Check sheet for the modelled part. Datum: model origin and axes. Units: mm. Give positions to 0.01 mm unless a question says otherwise; leave off trailing zeros. Loops run counter-clockwise (first coordinate to the right, second up) from the corner with the lowest first, then second, coordinate; pieces in that order, holes last.
```python
from build123d import *

# Parameters (mm, degrees)
F0_R     = 1.5
F0_R_2   = 1.25
F0_R_3   = 3.35
F1_DEPTH = 2.5


with BuildPart() as f1:
    # F0 (on Top) → F1 (new body)
    with BuildSketch(Plane.XY):
        with BuildLine():
            Line((-8.0347370397, 15.957047836), (-11, -56))
            Line((-11, -56), (-7.9966708881, -63.1295586577))
            ThreePointArc((-7.9966708881, -63.1295586577), (0, -68), (7.9966708881, -63.1295586577))
            Line((7.9966708881, -63.1295586577), (11, -56))
            Line((11, -56), (8.0347370397, 15.957047836))
            ThreePointArc((8.0347370397, 15.957047836), (8.1132286629, 16.7731349004), (8.4097212043, 17.5374981677))
            Line((8.4097212043, 17.5374981677), (12.5735371817, 25.0323669271))
            ThreePointArc((12.5735371817, 25.0323669271), (12.8772178164, 25.8277582971), (12.9452230888, 26.6764305791))
            Line((12.9452230888, 26.6764305791), (12.0626597761, 40.7974435824))
            ThreePointArc((12.0626597761, 40.7974435824), (11.8483082239, 41.738438851), (11.3462718477, 42.5626828443))
            Line((11.3462718477, 42.5626828443), (6.8979650397, 47.7523741204))
            ThreePointArc((6.8979650397, 47.7523741204), (5.8737656612, 48.5255386955), (4.6201952326, 48.8))
            Line((4.6201952326, 48.8), (-4.6201952326, 48.8))
            ThreePointArc((-4.6201952326, 48.8), (-5.8737656612, 48.5255386955), (-6.8979650397, 47.7523741204))
            Line((-6.8979650397, 47.7523741204), (-11.3462718477, 42.5626828443))
            ThreePointArc((-11.3462718477, 42.5626828443), (-11.8483082239, 41.738438851), (-12.0626597761, 40.7974435824))
            Line((-12.0626597761, 40.7974435824), (-12.9452230888, 26.6764305791))
            ThreePointArc((-12.9452230888, 26.6764305791), (-12.8772178164, 25.8277582971), (-12.5735371817, 25.0323669271))
            Line((-12.5735371817, 25.0323669271), (-8.4097212043, 17.5374981677))
            ThreePointArc((-8.4097212043, 17.5374981677), (-8.1132286629, 16.7731349004), (-8.0347370397, 15.957047836))
        make_face()
        with Locations((-6, -57.6)):
            Circle(F0_R, mode=Mode.SUBTRACT)
        with Locations((-6, -47.6)):
            Circle(F0_R, mode=Mode.SUBTRACT)
        with Locations((6, -57.6)):
            Circle(F0_R, mode=Mode.SUBTRACT)
        with Locations((6, -47.6)):
            Circle(F0_R, mode=Mode.SUBTRACT)
        with Locations((0, 1.25)):
            Circle(F0_R_2, mode=Mode.SUBTRACT)
        with Locations((0, 8.75)):
            Circle(F0_R_2, mode=Mode.SUBTRACT)
        with BuildLine():
            Line((-7.9549512883, 26.8285010896), (-5.6922095886, 29.0912427894))
            ThreePointArc((-5.6922095886, 29.0912427894), (-3.3587572106, 29.0912427894), (-3.3587572106, 26.7577904114))
            Line((-3.3587572106, 26.7577904114), (-5.6214989104, 24.4950487117))
            ThreePointArc((-5.6214989104, 24.4950487117), (-7.9549512883, 24.4950487117), (-7.9549512883, 26.8285010896))
        make_face(mode=Mode.SUBTRACT)
        with Locations((0, 32.45)):
            Circle(F0_R_3, mode=Mode.SUBTRACT)
        with BuildLine():
            Line((-5.6214989104, 40.4049512883), (-3.3587572106, 38.1422095886))
            ThreePointArc((-3.3587572106, 38.1422095886), (-3.3587572106, 35.8087572106), (-5.6922095886, 35.8087572106))
            Line((-5.6922095886, 35.8087572106), (-7.9549512883, 38.0714989104))
            ThreePointArc((-7.9549512883, 38.0714989104), (-7.9549512883, 40.4049512883), (-5.6214989104, 40.4049512883))
        make_face(mode=Mode.SUBTRACT)
        with BuildLine():
            Line((5.6214989104, 24.4950487117), (3.3587572106, 26.7577904114))
            ThreePointArc((3.3587572106, 26.7577904114), (3.3587572106, 29.0912427894), (5.6922095886, 29.0912427894))
            Line((5.6922095886, 29.0912427894), (7.9549512883, 26.8285010896))
            ThreePointArc((7.9549512883, 26.8285010896), (7.9549512883, 24.4950487117), (5.6214989104, 24.4950487117))
        make_face(mode=Mode.SUBTRACT)
        with BuildLine():
            Line((7.9549512883, 38.0714989104), (5.6922095886, 35.8087572106))
            ThreePointArc((5.6922095886, 35.8087572106), (3.3587572106, 35.8087572106), (3.3587572106, 38.1422095886))
            Line((3.3587572106, 38.1422095886), (5.6214989104, 40.4049512883))
            ThreePointArc((5.6214989104, 40.4049512883), (7.9549512883, 40.4049512883), (7.9549512883, 38.0714989104))
        make_face(mode=Mode.SUBTRACT)
    extrude(amount=F1_DEPTH)


solid = f1.part
```
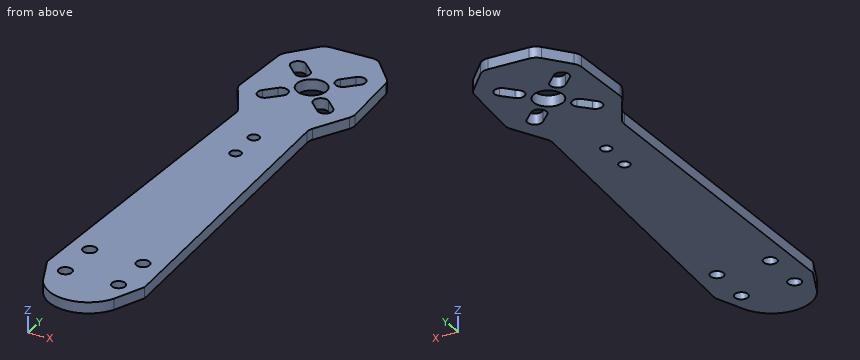
(1) Section check B-B on y = 31. Record the boundary of the cut face in (x, z) (3 decimals), plus the area to 3 significant figures.
(2) Gauge pin test, flat ends, axial feed: pin 1 Ø2.5 at (x, y) = (6, -47.6) entering from +Z; pin 2 Ø1.5 at (y, z) = (-49, 0.5) entering from -X; pin 3 Ø1 at (y, z) = (21, 1.5) entering from +X. Record the tip position at first contact, or that the pin passes through.
(3) Section check D-D on z = 1.55. Give the number of separate pieces and of enclosed holes in the cut face, plus the area to 3 significant figures.
(4) Section check C-C on y = -57.6. Record the boundary of the cut face in (x, z).
(5) Section check A-A on x = 0. Record the boundary of the cut face in (y, z), plus the area to 3 significant figures.
(6) Material ranges on line 1 (Y direction, x = 0, z = 0.85); line 2 (Y direction, x = -6.5, z = 1.6); line 3 (X direction, y = -46.5, z = 1.85), recorded low to high.
Computed values:
1. outline: (-12.675, 0) - (-3.02, 0) - (-3.02, 2.5) - (-12.675, 2.5) - close; (3.02, 0) - (12.675, 0) - (12.675, 2.5) - (3.02, 2.5) - close
1. area: 48.3 mm2
2. pin 1: passes through
2. pin 2: stops at x = -10.74
2. pin 3: stops at x = 10.61
3. separate pieces: 1
3. enclosed holes: 11
3. area: 2,140 mm2
4. outline: (-10.33, 0) - (-7.5, 0) - (-7.5, 2.5) - (-10.33, 2.5) - close; (-4.5, 0) - (4.5, 0) - (4.5, 2.5) - (-4.5, 2.5) - close; (7.5, 0) - (10.33, 0) - (10.33, 2.5) - (7.5, 2.5) - close
5. outline: (-68, 0) - (0, 0) - (0, 2.5) - (-68, 2.5) - close; (2.5, 0) - (7.5, 0) - (7.5, 2.5) - (2.5, 2.5) - close; (10, 0) - (29.1, 0) - (29.1, 2.5) - (10, 2.5) - close; (35.8, 0) - (48.8, 0) - (48.8, 2.5) - (35.8, 2.5) - close
5. area: 263 mm2
6. line 1: y = -68 to 0, 2.5 to 7.5, 10 to 29.1, 35.8 to 48.8
6. line 2: y = -65.22 to -59.01, -56.19 to -49.01, -46.19 to 24.04, 28.28 to 36.62, 40.86 to 48.14
6. line 3: x = -10.61 to -7.02, -4.98 to 4.98, 7.02 to 10.61
